CAD build for the part. Positions are in the model's coordinates, mm. A direction names the side the tool comes from. Give positions to 0.01 mm unless a question says otherwise; leave off trailing zeros. Write each loop counter-clockwise with the first axis right and the second up, starting at its lowest first coordinate (ties: lowest second). Pieces come first, ordered by that corner, then holes. Notation, with made-up numbers: (53.5, 21.5) - (60.5, 21.5) arc R31 cw to (60.5, 49.5) - close; hole circle Ø11 at (-13.5, -36). An arc over 180 degrees is marked (long way). Write item = value, one per line. Start each with the question number.
Autodesk Inventor part; units mm, degrees
ref_plane "YZ Plane" through (0, 0, 0) normal (1, 0, 0) x (0, 1, 0)
ref_plane "XZ Plane" through (0, 0, 0) normal (0, 1, 0) x (-1, 0, 0)
ref_plane "XY Plane" through (0, 0, 0) normal (0, 0, 1) x (1, 0, 0)
sketch "Sketch1" plane through (0, 0, 0) normal (0, 1, 0) x (-1, 0, 0)
  line L0 (0, 0) -> (0, -3)
  line L1 (0, -3) -> (15, -3)
  line L2 (17, -5) -> (17, -102.86)
  line L3 (0, 0) -> (18, 0)
  line L4 (20, -2) -> (20, -102.86)
  line L5 (20, -102.86) -> (17, -102.86)
  arc A0 (17, -5) -> (15, -3) centre (15, -5) ccw
  arc A1 (20, -2) -> (18, 0) centre (18, -2) ccw
  point P0 (17, -3)
  point P1 (20, 0)
  dimension "d0" = 3
  dimension "d1" = 17
  dimension "d2" = 99.86
  dimension "d3" = 20
  dimension "d4" = 2
extrude "Extrusion1" add sketch "Sketch1" along normal blind 14
sketch "Sketch2" plane through (0, 0, -3) normal (0, 0, -1) x (-1, 0, 0)
  point P0 (0, 0)
sketch "Sketch3" plane through (0, 0, -3) normal (0, 0, -1) x (-1, 0, 0)
  circle A0 centre (2.3646, 7) radius 1.5
  circle A1 centre (12.3646, 7) radius 1.5
  line L0 (0, 14) -> (15, 14)
  line L1 (0, 0) -> (15, 0)
  dimension "d7" = 3
  dimension "d8" = 3
  dimension "d9" = 14
  dimension "d10" = 7
  dimension "d11" = 10
hole "Hole1" at (-2.3646, 7, -3) at (-12.3646, 7, -3) direction (0, 0, 1) diameter 2.459 depth 8.8 tip angle 118
sketch "Sketch4" plane through (-20, 0, -102.86) normal (-1, 0, 0) x (0, 0, 1)
  line L0 (10, 12.5) -> (37.5, 12.5)
  line L1 (37.5, 12.5) -> (37.5, 1.5)
  line L2 (37.5, 1.5) -> (10, 1.5)
  line L3 (10, 1.5) -> (10, 12.5)
  line L4 (0, 14) -> (100.86, 14)
  line L5 (0, 0) -> (100.86, 0)
  line L6 (0, 0) -> (0, 14)
  circle A0 centre (7, 7) radius 1.5
  circle A1 centre (40.32, 7) radius 1.5
  point P0 (102.86, 0)
  dimension "d19" = 27.5
  dimension "d20" = 11
  dimension "d21" = 14
  dimension "d22" = 1.5
  dimension "d23" = 10
  dimension "d24" = 3
  dimension "d25" = 3
  dimension "d26" = 33.32
  dimension "d29" = 7
hole "Hole2" at (-20, 7, -62.54) at (-20, 7, -95.86) direction (1, 0, 0) diameter 2.459 depth 8.8 tip angle 118
extrude "Extrusion2" cut sketch "Sketch4" against normal blind 14 contours L0 L1 L2 L3
equation "\"d10\" = 0.5 * d9"
equation "\"d22\" = -0.5 * d20 + 0.5 * d21"
properties part number "płytka złącza"
1. Mould opens along Y. For faces 4 (the cylindrical face through (-18.479, 7.471, -94.724)), 5 (the flat face through (-19, 7, -92.86)), 6 (the flat face through (-9, 7, 0)), 7 (the flat face through (-18, 14, -44)) say: +Y half, -Y half, draft (parallel to the pull), parting line (faces both ways), or undercut.
2. Tool access for faces 1 (the flat face through (-20, 7, -41)), 2 (the flat face through (-19, 1.5, -79)), 3 (the flat face through (-7, 7, -3)): list every direction of +Z, -Z, +X, -X, +Y, -Y with a clear straight run to the whole face (end or side of a thin tool).
3. Cut at A-A (z = -62.54). Give the cut face in (x, y), then the cut area to 3 significant figures.
4. Pin check, flat tips, straight feed: pin 1 Ø8 at (x, z) = (-14.5, -25.5) entering from +Y; pin 2 Ø1 at (x, y) = (-4.5, 12) entering from -Z; pin 3 Ø6 at (y, z) = (5, -61) entering from +X. Stop position of each tip, or through.
5. Cut at C-C (z = -11.5). Give the cut face in (x, y), then the cut area to 3 significant figures.
6. Wall check: line 1 along X through (y, z) = (7, -2); line 2 along Z through (x, y) = (-18.8, 7); line 3 along X through (y, z) = (7, -0.7). Give the ranges that are in metal, low to high.
7. Cut at B-B (y = 10.5). Give the cut face in (x, z).
8. Cut at D-D (x = -5.75). Give the cut face in (y, z), then the cut area to 3 significant figures.
Output:
q1.face_4 = undercut
q1.face_5 = undercut
q1.face_6 = draft
q1.face_7 = +Y half
q2.face_1 = +Z, -Z, -X, +Y, -Y
q2.face_2 = +X, -X
q2.face_3 = -Z, +X, +Y, -Y
q3.outline = (-20, 0) - (-17, 0) - (-17, 5.77) - (-20, 5.77) - close; (-20, 8.23) - (-17, 8.23) - (-17, 14) - (-20, 14) - close
q3.area = 34.6 mm2
q4.pin_1 = 14
q4.pin_2 = -3
q4.pin_3 = -17
q5.outline = (-20, 0) - (-17, 0) - (-17, 14) - (-20, 14) - close
q5.area = 42.0 mm2
q6.line_1 = -20 to -13.59, -11.14 to -3.59, -1.14 to 0
q6.line_2 = -102.86 to -97.09, -94.63 to -92.86, -65.36 to -63.77, -61.31 to -0.17
q6.line_3 = -19.52 to -13.59, -11.14 to -3.59, -1.14 to 0
q7.outline = (-20, -102.86) - (-17, -102.86) - (-17, -92.86) - (-20, -92.86) - close; (-20, -65.36) - (-17, -65.36) - (-17, -5) arc R2 cw to (-15, -3) - (0, -3) - (0, 0) - (-18, 0) arc R2 ccw to (-20, -2) - close
q8.outline = (0, -3) - (14, -3) - (14, 0) - (0, 0) - close
q8.area = 42.0 mm2
